Check sheet for the modelled part. Datum: model origin and axes. Units: mm. A direction names the side the tool comes from. Give positions to 0.01 mm unless a question says otherwise; leave off trailing zeros. Loops run counter-clockwise (first coordinate to the right, second up) from the corner with the lowest first, then second, coordinate; pieces in that order, holes last. Notation, with made-up numbers: (-12.5, 81.5) - (4.5, 81.5) arc R16 cw to (4.5, 102.5) - close; hole circle Ø3 at (62, 27.25). An arc over 180 degrees is marked (long way). Answer in a Markdown table with one row per item. Add a question column.
(1) Thickness scan on L1, parallel to Z at x = 27.5, y = 8; L2, parallel to Y at x = 1.35, z = 10; L3, parallel to X at y = 5.75, z = 10. Record the ranges inside material, lowest first.
(2) Sectioned sample at D-D on y = 36. Enter the section's corners in (x, z).
(3) Set-up check for faces 4 (the face through (22.146, 5.028, 10.676)), 5 (the face through (4, 22.3, 11.2)): record each of +Z, -Z, +X, -X, +Y, -Y from which the full face is reachable in a straight line by a thin tool's end or side.
(4) Sectioned sample at B-B on x = 20. Enter the section's corners in (y, z).
(5) Draft check along Y on faces 1 (the face through (19.7, 3, 7.6)), 2 (the face through (40, 5, 10)), 3 (the face through (1.972, 22.146, 10.676)). Enter one of: released by +Y, released by -Y, zero draft, split by the parting line, or undercut.
(6) Sectioned sample at C-C on z = 13.25. Enter the section's corners in (x, y), then the cut area to 3 significant figures.
(7) Sectioned sample at A-A on z = 10. Enter the section's corners in (x, y).
(8) Go/stop test with flat-tipped pins: P1, Ø12, axis at x = 33.5, z = 5, coming from the +Y side; P2, Ø5, axis at y = 20, z = 10, coming from the +X side. Record where each tip stops, or that it passes through.
from build123d import *

# Parameters (mm, degrees)
CYLINDER001_R     = 40
CYLINDER001_DEPTH = 20
CYLINDER002_R     = 2.25
CYLINDER002_DEPTH = 20
ARRAY002_COUNT    = 2
ARRAY002_ANGLE    = 90
BOX002_W          = 40
BOX002_H          = 37
BOX002_DEPTH      = 12
BOX001_W          = 40
BOX001_H          = 37
BOX001_DEPTH      = 20


with BuildPart() as cylinder001:
    # Cylinder001 → Cylinder001 (new body)
    with BuildSketch(Plane(origin=(43, 47, 0), x_dir=(1, 0, 0), z_dir=(0, 0, 1))):
        Circle(CYLINDER001_R)
    extrude(amount=CYLINDER001_DEPTH)


with BuildPart() as array002:
    # Cylinder002 → Cylinder002 (new body)
    with BuildSketch(Plane(origin=(20, 10, 10), x_dir=(1, 0, 0), z_dir=(0, -1, 0))):
        Circle(CYLINDER002_R)
    extrude(amount=CYLINDER002_DEPTH)

    # Array002: Array002 ×2 about axis
    array002_axis = Axis((0, 0, 0), (0, 0, 1))


with BuildPart() as array002_1:
    add(array002.part)
    for i in range(1, ARRAY002_COUNT):
        add(array002.part.rotate(array002_axis, i * ARRAY002_ANGLE / (ARRAY002_COUNT - 1)))


with BuildPart() as fusion:
    # Box002 → Box002 (new body)
    with BuildSketch(Plane(origin=(4, 7, 4), x_dir=(1, 0, 0), z_dir=(0, 0, 1))):
        with Locations((20, 18.5)):
            Rectangle(BOX002_W, BOX002_H)
    extrude(amount=BOX002_DEPTH)

    # Fusion: union Cylinder001, Array002
    add(cylinder001.part)
    add(array002_1.part)


with BuildPart() as cut001:
    # Box001 → Box001 (new body)
    with BuildSketch(Plane(origin=(0, 3, 0), x_dir=(1, 0, 0), z_dir=(0, 0, 1))):
        with Locations((20, 18.5)):
            Rectangle(BOX001_W, BOX001_H)
    extrude(amount=BOX001_DEPTH)

    # Cut001: cut Fusion
    add(fusion.part, mode=Mode.SUBTRACT)


solid = cut001.part
Reply:
| question | item | result |
|---|---|---|
| 1 | L1 | 0 to 4, 16 to 20 |
| 1 | L2 | 3 to 17.75, 22.25 to 40 |
| 1 | L3 | 0 to 17.75, 22.25 to 40 |
| 2 | outline | (0, 0) - (4.54, 0) - (4.54, 4) - (4, 4) - (4, 16) - (4.54, 16) - (4.54, 20) - (0, 20) - close |
| 3 | face 4 | +Y, -Y |
| 3 | face 5 | +X, +Y |
| 4 | outline | (3, 0) - (14.27, 0) - (14.27, 4) - (7, 4) - (7, 7.75) - (3, 7.75) - close; (3, 12.25) - (7, 12.25) - (7, 16) - (14.27, 16) - (14.27, 20) - (3, 20) - close |
| 5 | face 1 | released by -Y |
| 5 | face 2 | zero draft |
| 5 | face 3 | undercut |
| 6 | outline | (0, 3) - (40, 3) - (40, 7) - (4, 7) - (4, 38.11) arc R40 cw to (3.62, 40) - (0, 40) - close |
| 6 | area | 292 mm^2 |
| 7 | outline | (0, 3) - (17.75, 3) - (17.75, 7) - (4, 7) - (4, 17.75) - (0, 17.75) - close; (0, 22.25) - (4, 22.25) - (4, 38.11) arc R40 cw to (3.62, 40) - (0, 40) - close; (22.25, 3) - (40, 3) - (40, 7) - (22.25, 7) - close |
| 8 | P1 | y = 10.09 |
| 8 | P2 | x = 4 |
